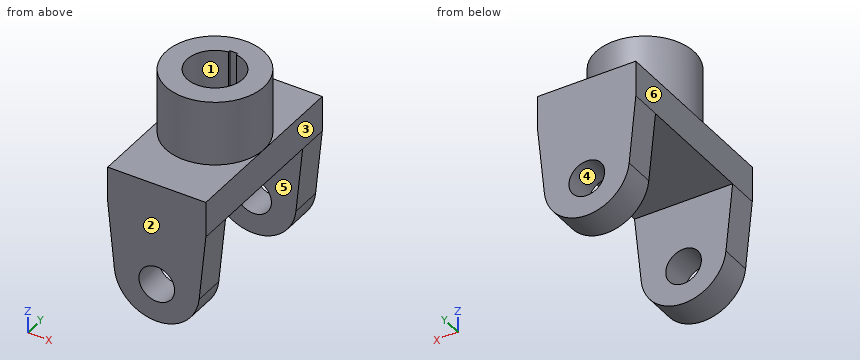
```python
from build123d import *

# Parameters (mm, degrees)
SKETCH2_W           = 88
SKETCH2_H           = 32
SKETCH2_R           = 16
BOSS_EXTRUDE2_DEPTH = 166
SKETCH5_W           = 94.38952736
SKETCH5_H           = 110
CUT_EXTRUDE1_DEPTH  = 166
SKETCH6_R           = 44
BOSS_EXTRUDE4_DEPTH = 58


with BuildPart() as part:
    # Sketch2 → Boss-Extrude2 (new body)
    # profile 1 of 2: a face of its own
    with BuildSketch(Plane(origin=(0, 0, 0), x_dir=(1, 0, 0), z_dir=(0, 1, 0))):
        with Locations((44, 16)):
            Rectangle(SKETCH2_W, SKETCH2_H)
    # profile 2 of 2: a face of its own
    with BuildSketch(Plane(origin=(0, 0, 0), x_dir=(1, 0, 0), z_dir=(0, 1, 0))):
        with BuildLine():
            ThreePointArc((6, 92), (44, 126.38952736), (82, 92))
            Line((82, 92), (88, 32))
            Line((88, 32), (0, 32))
            Line((0, 32), (6, 92))
        make_face()
        with Locations(Location((44, 92, 0), (0, 0, 270))):
            Circle(SKETCH2_R, mode=Mode.SUBTRACT)
    extrude(amount=BOSS_EXTRUDE2_DEPTH)

    # Sketch5 → Cut-Extrude1 (cut)
    with BuildSketch(Plane(origin=(0, 0, 0), x_dir=(0, 0, -1), z_dir=(1, 0, 0))):
        with Locations((79.19476368, 83)):
            Rectangle(SKETCH5_W, SKETCH5_H)
    extrude(amount=CUT_EXTRUDE1_DEPTH, mode=Mode.SUBTRACT)

    # Sketch6 → Boss-Extrude4 (add)
    with BuildSketch(Plane.XY):
        with Locations((44, 83)):
            Circle(SKETCH6_R)
        with BuildLine():
            Line((40.50858553, 107.755), (40.50858553, 109.755))
            Line((40.50858553, 109.755), (47.50858553, 109.755))
            Line((47.50858553, 109.755), (47.50858553, 107.752572141))
            ThreePointArc((47.50858553, 107.752572141), (43.991329074, 58.000001504), (40.50858553, 107.755))
        make_face(mode=Mode.SUBTRACT)
    extrude(amount=BOSS_EXTRUDE4_DEPTH)


solid = part.part
```
Geometry check sheet. Reference: the model listing, model coordinates, mm. Face numbers are marked on the shaded views. A direction names the side the tool comes from. Coordinates: 2 decimals unless noted, no trailing zeros. Order: outer loops, then holes, each group sorted by start corner. A loop starts at its lowest first (then second) coordinate and runs counter-clockwise, first axis right, second up. Notation, with made-up numbers: (73.25, 69.25) - (79.25, 69.25) arc R8 ccw to (79.25, 84.25) - close; hole circle Ø5 at (48, 42). An arc over 180 degrees is marked (long way). Use one line per item in the form item = value.
1. Section check A-A (x = 44). Record the boundary of the cut face in (y, z) (3 decimals), then the cut area to 3 significant figures.
Here are the results:
outline = (0, -126.39) - (28, -126.39) - (28, -108) - (0, -108) - close; (0, -76) - (28, -76) - (28, -32) - (138, -32) - (138, -76) - (166, -76) - (166, 0) - (127, 0) - (127, 58) - (109.755, 58) - (109.755, 0) - (58, 0) - (58, 58) - (39, 58) - (39, 0) - (0, 0) - close; (138, -126.39) - (166, -126.39) - (166, -108) - (138, -108) - close
area = 10,900 mm²
2. Section check C-C (y = 100). Record the boundary of the cut face in (x, z).
Here are the results:
outline = (0, -32) - (88, -32) - (88, 0) - (84.58, 0) - (84.58, 58) - (62.33, 58) - (62.33, 0) - (25.67, 0) - (25.67, 58) - (3.42, 58) - (3.42, 0) - (0, 0) - close
3. Draft check along X on the marked faces 1, 2, 3 and 4. Enter one of: pulls with the +X half, pulls with the -X half, needs draft (parallel to the pull), parting line crosses it, or undercut.
Here are the results:
face_1 = undercut
face_2 = needs draft
face_3 = pulls with the +X half
face_4 = undercut
4. Access from +Z, -Z, +X, -X, +Y, -Y to the whole of each face (thin tool, end or side, straight path). Record for the marked faces 5 and 6.
Here are the results:
face_5 = -Z, +X, -X
face_6 = +Z, -Z, -X, +Y, -Y
5. Section check B-B (z = 43). Record the boundary of the cut face in (x, y) (3 decimals).
Here are the results:
outline = circle Ø88 at (44, 83); hole (40.509, 107.755) arc R25 ccw (long way) to (47.509, 107.753) - (47.509, 109.755) - (40.509, 109.755) - close
6. Section check D-D (x = 15). Record the boundary of the cut face in (y, z).
Here are the results:
outline = (0, -113.05) - (28, -113.05) - (28, -32) - (138, -32) - (138, -113.05) - (166, -113.05) - (166, 0) - (116.09, 0) - (116.09, 58) - (49.91, 58) - (49.91, 0) - (0, 0) - close
7. Scan lines: line 1 (X direction, y = 17.5, z = -92); line 2 (Y direction, x = 7, z = -48.5); line 3 (Z direction, x = 44, y = 11). Record each from-to range of solid material in increasing order.
Here are the results:
line_1 = 6 to 28, 60 to 82
line_2 = 0 to 28, 138 to 166
line_3 = -126.39 to -108, -76 to 0
8. Gauge pin test, flat ends, axial feed: pin 1 (8 mm diameter, centred on x = 20.5, y = 79, fed in from -Z); pin 2 (1.5 mm diameter, centred on x = 11.5, y = 32, fed in from +Z); pin 3 (0.6 mm diameter, centred on y = 108.5, z = 41, fed in from +X). Record the tip position at first contact, or that the pin passes through.
Here are the results:
pin_1 = -32
pin_2 = 0
pin_3 = 80.07
